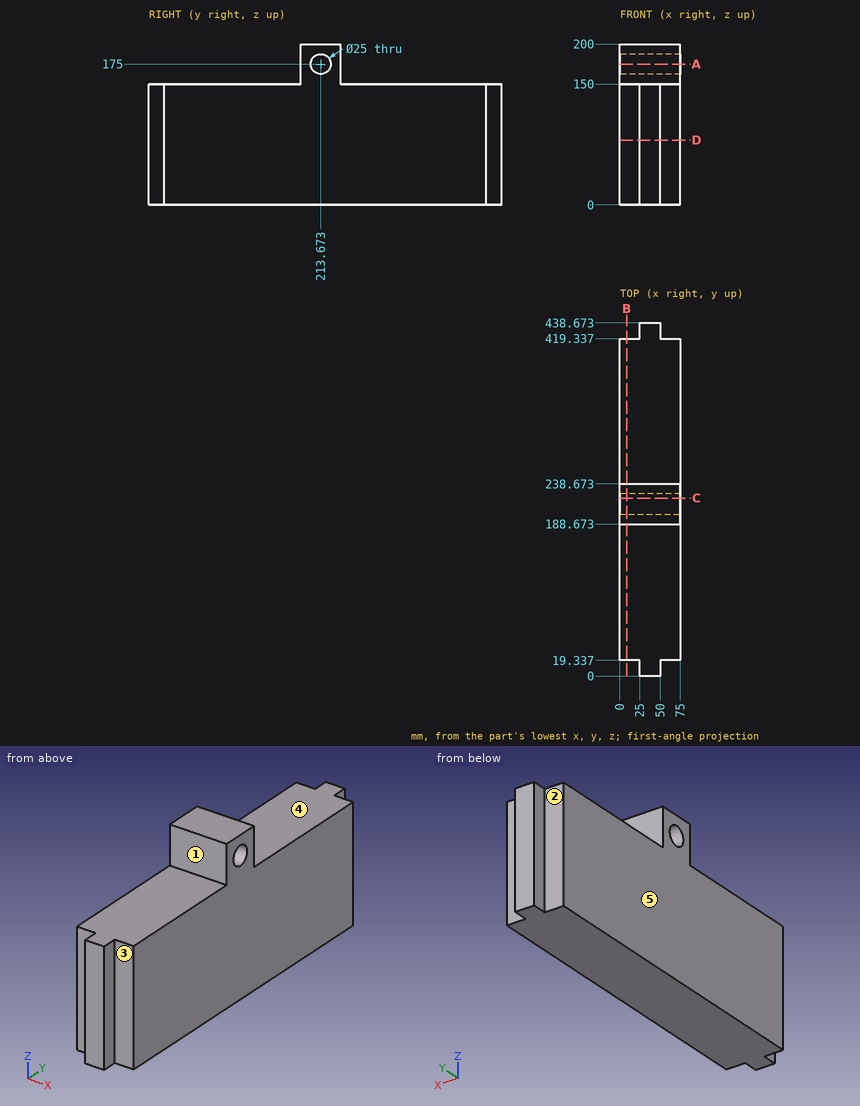
Geometry: see drawing. Coordinates: mm, zero at the bounding-box minimum. A direction names the side the tool comes from. Give positions to 0.01 mm unless a question says otherwise; leave off trailing zeros. Loops run counter-clockwise (first coordinate to the right, second up) from the corner with the lowest first, then second, coordinate; pieces in that order, holes last. Notation, with made-up numbers: (37, 46.25) - (48, 46.25) arc R23 cw to (48, 65.25) - close; hole circle Ø1 at (37.25, 30.25). An arc over 180 degrees is marked (long way). Answer as CSV lines item,"result". Start each with the question number.
1. Section C-C, the plane y = 221. Return loops of the section in (x, z).
2. Section A-A, the plane z = 175. Return loops of the section in (x, y).
3. Pin query (flat end, axial travel): P1, Ø6, axis at y = 11.5, z = 86, coming from the +X side; P2, Ø6, axis at x = 40.5, z = 171, coming from the +Y side; P3, Ø5, axis at x = 59, z = 132.5, coming from the +Y side. Return the tip coordinate at first contact, or that it passes through.
4. Reachability of the marked faces 1, 2, 3, 4 and 5 from +Z, -Z, +X, -X, +Y, -Y: full face, straight path, thin tool, end or side. Return the list, or none.
5. Section B-B, the plane x = 8.5. Return loops of the section in (y, z).
6. Ray query, L1, parallel to Y at x = 6, z = 65; L2, parallel to Z at x = 46.5, y = 222.5; L3, parallel to Y at x = 34, z = 183.5 (1 decimal). Return the intervals inside material, ascending.
7. Section D-D, the plane z = 80.5. Return loops of the section in (x, y), plus the area to 3 significant figures.
Answers:
1,outline,"(0, 0) - (75, 0) - (75, 164.87) - (0, 164.87) - close; (0, 185.13) - (75, 185.13) - (75, 200) - (0, 200) - close"
2,outline,"(0, 188.67) - (75, 188.67) - (75, 201.17) - (0, 201.17) - close; (0, 226.17) - (75, 226.17) - (75, 238.67) - (0, 238.67) - close"
3,P1,"stops at x = 50"
3,P2,"stops at y = 238.67"
3,P3,"stops at y = 419.34"
4,face 1,"+Z, +X, -X, -Y"
4,face 2,"+Z, -Z, -X, +Y"
4,face 3,"+Z, -Z, +X, -Y"
4,face 4,"+Z, +X, -X, +Y"
4,face 5,"+Z, -Z, -X, +Y, -Y"
5,outline,"(19.34, 0) - (419.34, 0) - (419.34, 150) - (238.67, 150) - (238.67, 200) - (188.67, 200) - (188.67, 150) - (19.34, 150) - close; hole circle Ø25 at (213.67, 175)"
6,L1,"y = 19.34 to 419.34"
6,L2,"z = 0 to 166.15, 183.85 to 200"
6,L3,"y = 188.7 to 204.5, 222.8 to 238.7"
7,outline,"(0, 19.34) - (25, 19.34) - (25, 0) - (50, 0) - (50, 19.34) - (75, 19.34) - (75, 419.34) - (50, 419.34) - (50, 438.67) - (25, 438.67) - (25, 419.34) - (0, 419.34) - close"
7,area,"31,000 mm2"
